Design review of the part built by this model. Coordinates are the model's own, in mm. Coordinates: 2 decimals unless noted, no trailing zeros. Loops run counter-clockwise (first coordinate to the right, second up) from the corner with the lowest first, then second, coordinate; pieces in that order, holes last. Notation, with made-up numbers: (23.5, -17) - (74.5, -17) arc R13 cw to (74.5, -13) - close; hole circle Ø1 at (18.25, 49). An arc over 180 degrees is marked (long way). Answer in a Markdown table with one row per item. Add a question column.
(1) We need section C-C, the plane y = -8. Write out the cut boundary in (x, z), plus the area to 3 significant figures.
(2) The part is to be moulded in two halves that separate along Z. For faces 1 (the face through (-5.807, 6.235, -4.444)), 2 (the face through (0, 10, -5)), 3 (the face through (-7, 0, -10)), 4 (the face through (-4.53, -6.15, -4.92)), say which applies: released by +Z, released by -Z, zero draft, split by the parting line, or undercut.
(3) We need section B-B, the plane z = -4. Write out the cut boundary in (x, y) (3 decimals), plus the area to 3 significant figures.
(4) We need section A-A, the plane x = -3.25. Write out the cut boundary in (y, z).
(5) To check wall thickness, follow L1, parallel to Z at x = -3.5, y = 8; L2, parallel to Y at x = -8.25, z = -5; L3, parallel to Y at x = -5.75, z = -5. State the ranges of each line that lie inside material, in increasing order. Write a range as [from, to].
(6) We need section D-D, the plane x = -1. Write out the cut boundary in (y, z).
(7) Clearance check with flat-ended pins moving along their axes: pin 1 (3 mm diameter, centred on x = -10, z = -2, fed in from -Y); pin 2 (6 mm diameter, centred on y = 0.5, z = -7, fed in from -X); pin 3 (1.5 mm diameter, centred on x = -11, z = -9, fed in from +Y); pin 4 (3 mm diameter, centred on y = 4.5, z = -4, fed in from -X). State where each tip first meets the part, or that it passes through.
from build123d import *

# Parameters (mm, degrees)
F0_W        = 6.7956063077
F0_H        = 13
F0_H_2      = 6.5
F0_W_2      = 6.2043936923
F1_DEPTH    = 10
F2_R        = 1.85
F3_DEPTH    = 13
F4_T1_DEPTH = 75


# Not quite as in the source:
# - a fillet or chamfer that OpenCascade refuses, or shapes differently, is made with other operations: its cross-section is extruded or revolved along the edge and cut away or added
# - a feature names something its author has since deleted; it is built from what else it names


with BuildPart() as f1:
    # F0 (on Top) → F1 (new body)
    with BuildSketch(Plane.XY):
        with BuildLine():
            Line((0, 6.5), (-6.2043936923, 6.5))
            Line((-6.2043936923, 6.5), (-6.2043936923, -6.5))
            Line((-6.2043936923, -6.5), (0, -6.5))
            Line((0, -6.5), (0, -3.825))
            ThreePointArc((0, -3.825), (-3.825, 0), (0, 3.825))
            Line((0, 3.825), (0, 6.5))
        make_face()
        with Locations((-9.6021968462, 0)):
            Rectangle(F0_W, F0_H)
        with Locations((-9.6021968462, 9.75)):
            Rectangle(F0_W, F0_H_2)
        with Locations((-3.1021968462, 9.75)):
            Rectangle(F0_W_2, F0_H_2)
        Polygon((-6.2043936923, -6.5), (-13, -6.5), (-13, -13), (0, -13), (0, -6.5), align=None)
    extrude(amount=-F1_DEPTH)

    # F2 (on face) → F3 (cut, through all)
    with BuildSketch(Plane(origin=(-13, 0, 0), x_dir=(0, -1, 0), z_dir=(-1, 0, 0))):
        with Locations((-8, -5)):
            Circle(F2_R)
        with Locations((8, -5)):
            Circle(F2_R)
    extrude(amount=-F3_DEPTH, mode=Mode.SUBTRACT)

    # F4: fillet of radius 13 on 2 edges, made by hand

    # F4_s2 → F4_t1 (cut)
    with BuildSketch(Plane.XY.offset(-42.5)):
        with BuildLine():
            ThreePointArc((0, 13), (-9.1923881554, 9.1923881554), (-13, 0))
            Line((-13, 0), (-13, 13))
            Line((-13, 13), (0, 13))
        make_face()
        with BuildLine():
            ThreePointArc((0, -13), (-9.1923881554, -9.1923881554), (-13, 0))
            Line((-13, 0), (-13, -13))
            Line((-13, -13), (0, -13))
        make_face()
    extrude(amount=F4_T1_DEPTH, mode=Mode.SUBTRACT)


solid = f1.part
Responses:
| question | item | result |
|---|---|---|
| 1 | outline | (-10.25, -10) - (0, -10) - (0, -6.85) - (-10.25, -6.85) - close; (-10.25, -3.15) - (0, -3.15) - (0, 0) - (-10.25, 0) - close |
| 1 | area | 64.6 mm2 |
| 2 | face 1 | undercut |
| 2 | face 2 | zero draft |
| 2 | face 3 | released by -Z |
| 2 | face 4 | undercut |
| 3 | outline | (-11.291, -6.444) - (0, -6.444) - (0, -3.825) arc R3.825 cw to (0, 3.825) - (0, 6.444) - (-11.291, 6.444) arc R13 ccw to start; (-8.813, -9.556) arc R13 ccw to (0, -13) - (0, -9.556) - close; (-8.813, 9.556) - (0, 9.556) - (0, 13) arc R13 ccw to start |
| 3 | area | 179 mm2 |
| 4 | outline | (-12.59, -10) - (-2.02, -10) - (-2.02, 0) - (-12.59, 0) - close; (2.02, -10) - (12.59, -10) - (12.59, 0) - (2.02, 0) - close; hole circle Ø3.7 at (-8, -5); hole circle Ø3.7 at (8, -5) |
| 5 | L1 | z = [-10, -6.85], [-3.15, 0] |
| 5 | L2 | y = [-10.05, -9.85], [-6.15, 6.15], [9.85, 10.05] |
| 5 | L3 | y = [-11.66, -9.85], [-6.15, 6.15], [9.85, 11.66] |
| 6 | outline | (-12.96, -10) - (-3.69, -10) - (-3.69, 0) - (-12.96, 0) - close; (3.69, -10) - (12.96, -10) - (12.96, 0) - (3.69, 0) - close; hole circle Ø3.7 at (-8, -5); hole circle Ø3.7 at (8, -5) |
| 7 | pin 1 | stops at y = -9.84 |
| 7 | pin 2 | stops at x = -13 |
| 7 | pin 3 | stops at y = 8 |
| 7 | pin 4 | stops at x = -12.65 |
